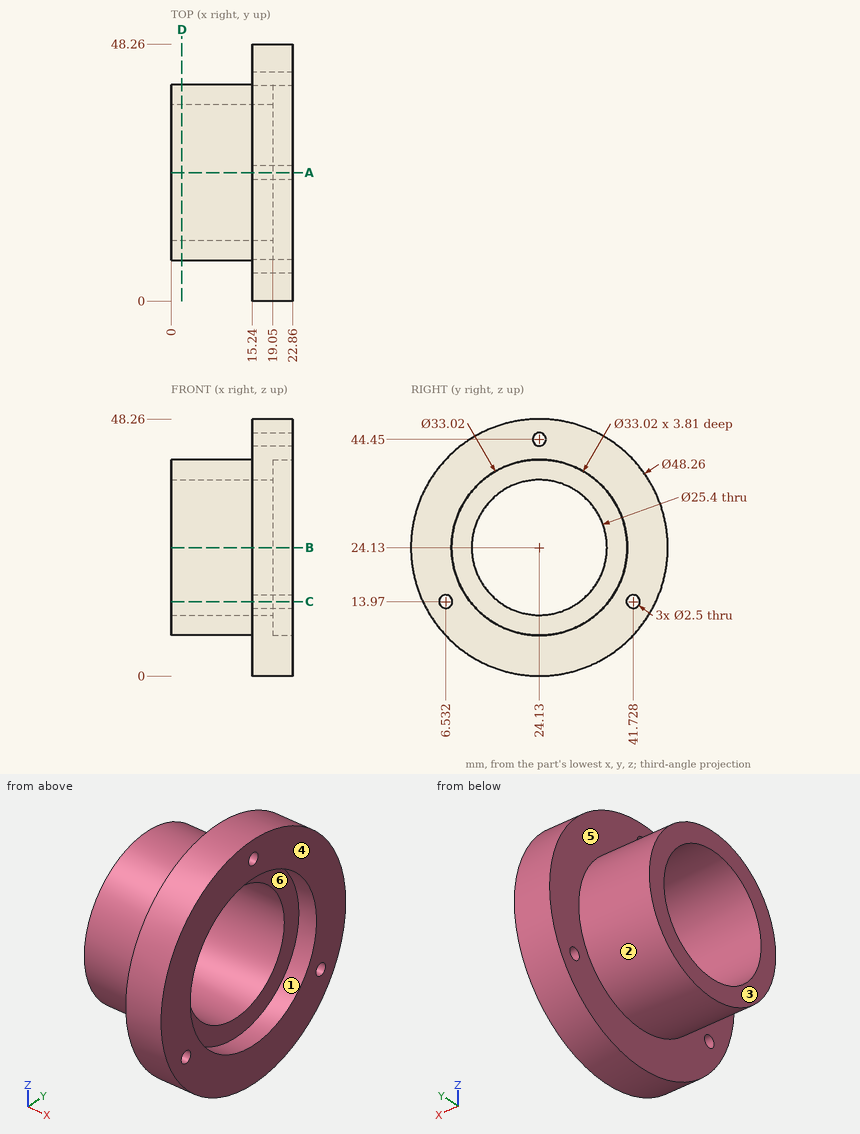
Job drawing, mm, ordinate dimensions from the low corner. One solid piece. A direction names the side the tool comes from. Round coordinates to 2 decimals unless told otherwise and drop trailing zeros. Order: outer loops, then holes, each group sorted by start corner. A loop starts at its lowest first (then second) coordinate and runs counter-clockwise, first axis right, second up. Notation, with made-up numbers: (45, -5.5) -> (82, -5.5) arc R36 ccw to (82, 29.5) -> close; hole circle Ø9 at (69, 67). An arc over 180 degrees is marked (long way). Answer in a Markdown table with one row per item.
1) Pin check, flat tips, straight feed: P1, Ø1, axis at x = 19.5, y = 38.5, coming from the -Z side (1 decimal); P2, Ø10, axis at x = 11.5, z = 20.5, coming from the -Y side; P3, Ø3, axis at y = 41.73, z = 13.97, coming from the -X side. Stop position of each tip, or through.
Values:
| item | result |
|---|---|
| P1 | z = 4.4 |
| P2 | y = 0 |
| P3 | x = 15.24 |
2) Which spindle directions (+Z, -Z, +X, -X, +Y, -Y) get a long thin tool onto all of the face, cutting with end or side? Do the marked faces 4, 5 and 6. Say none if no direction does.
Values:
| item | result |
|---|---|
| face 4 | +Z, -Z, +X, +Y, -Y |
| face 5 | -X |
| face 6 | +X |
3) Band-saw the part on C-C on z = 13.97. Give the cut face in (x, y), and give its area (3 significant figures).
Values:
| item | result |
|---|---|
| outline | (0, 11.12) -> (15.24, 11.12) -> (15.24, 7.78) -> (22.86, 7.78) -> (22.86, 11.12) -> (19.05, 11.12) -> (19.05, 16.51) -> (0, 16.51) -> close; (0, 31.75) -> (19.05, 31.75) -> (19.05, 37.14) -> (22.86, 37.14) -> (22.86, 40.48) -> (15.24, 40.48) -> (15.24, 37.14) -> (0, 37.14) -> close; (15.24, 2.24) -> (22.86, 2.24) -> (22.86, 5.28) -> (15.24, 5.28) -> close; (15.24, 42.98) -> (22.86, 42.98) -> (22.86, 46.02) -> (15.24, 46.02) -> close |
| area | 303 mm2 |
4) Band-saw the part on B-B on z = 24.13. Give the cut face in (x, y), and give its area (3 significant figures).
Values:
| item | result |
|---|---|
| outline | (0, 7.62) -> (15.24, 7.62) -> (15.24, 0) -> (22.86, 0) -> (22.86, 7.62) -> (19.05, 7.62) -> (19.05, 11.43) -> (0, 11.43) -> close; (0, 36.83) -> (19.05, 36.83) -> (19.05, 40.64) -> (22.86, 40.64) -> (22.86, 48.26) -> (15.24, 48.26) -> (15.24, 40.64) -> (0, 40.64) -> close |
| area | 261 mm2 |
5) Mould opens along Y. For the marked faces 1, 2 and 3 say: released by +Y, released by -Y, zero draft, split by the parting line, or undercut.
Values:
| item | result |
|---|---|
| face 1 | undercut |
| face 2 | split by the parting line |
| face 3 | zero draft |
6) Wall check: L1, parallel to Z at x = 21.2, y = 24.13; L2, parallel to Z at x = 12.25, y = 24.13; L3, parallel to X at y = 11, z = 21. Give the ranges that are in metal, low to high.
Values:
| item | result |
|---|---|
| L1 | 0 to 7.62, 40.64 to 43.2, 45.7 to 48.26 |
| L2 | 7.62 to 11.43, 36.83 to 40.64 |
| L3 | 0 to 19.05 |
7) Band-saw the part on A-A on y = 24.13. Give the cut face in (x, z).
Values:
| item | result |
|---|---|
| outline | (0, 7.62) -> (15.24, 7.62) -> (15.24, 0) -> (22.86, 0) -> (22.86, 7.62) -> (19.05, 7.62) -> (19.05, 11.43) -> (0, 11.43) -> close; (0, 36.83) -> (19.05, 36.83) -> (19.05, 40.64) -> (22.86, 40.64) -> (22.86, 43.2) -> (15.24, 43.2) -> (15.24, 40.64) -> (0, 40.64) -> close; (15.24, 45.7) -> (22.86, 45.7) -> (22.86, 48.26) -> (15.24, 48.26) -> close |
8) Band-saw the part on D-D on x = 2. Give the cut face in (y, z).
Values:
| item | result |
|---|---|
| outline | circle Ø33.02 at (24.13, 24.13); hole circle Ø25.4 at (24.13, 24.13) |
